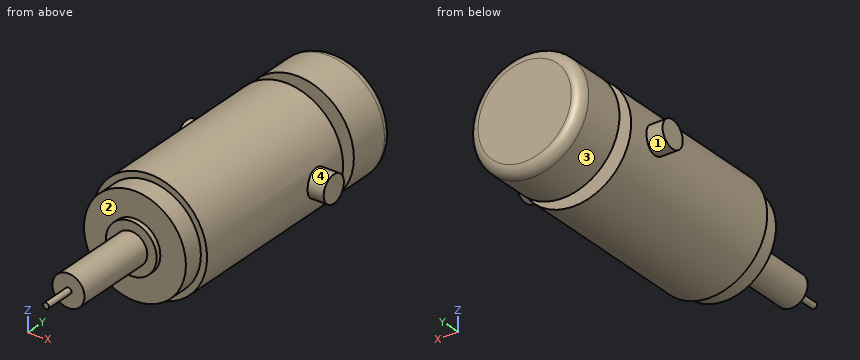
```python
from build123d import *

# Parameters (mm, degrees)
SKETCH1_R           = 28.5
BOSS_EXTRUDE1_DEPTH = 45.5
SKETCH4_R           = 25.4
BOSS_EXTRUDE4_DEPTH = 10
SKETCH5_R           = 12.65
BOSS_EXTRUDE5_DEPTH = 2.5
SKETCH2_R           = 8
BOSS_EXTRUDE2_DEPTH = 42
SKETCH6_R           = 4
BOSS_EXTRUDE6_DEPTH = 33
SKETCH7_R           = 28.25
BOSS_EXTRUDE7_DEPTH = 25.5
FILLET1_R           = 5
SKETCH3_R           = 1.5
BOSS_EXTRUDE3_DEPTH = 15
SKETCH8_R           = 6.75
BOSS_EXTRUDE8_DEPTH = 36.5


with BuildPart() as part:
    # Sketch1 → Boss-Extrude1 (new body, symmetric)
    with BuildSketch(Plane(origin=(0, 0, 0), x_dir=(1, 0, 0), z_dir=(0, 1, 0))):
        Circle(SKETCH1_R)
    extrude(amount=BOSS_EXTRUDE1_DEPTH, both=True)

    # Sketch4 → Boss-Extrude4 (add)
    with BuildSketch(Plane.XZ.offset(45.5)):
        Circle(SKETCH4_R)
    extrude(amount=BOSS_EXTRUDE4_DEPTH)

    # Sketch5 → Boss-Extrude5 (add)
    with BuildSketch(Plane.XZ.offset(55.5)):
        Circle(SKETCH5_R)
    extrude(amount=BOSS_EXTRUDE5_DEPTH)

    # Sketch2 → Boss-Extrude2 (add)
    with BuildSketch(Plane.XZ.offset(58)):
        Circle(SKETCH2_R)
    extrude(amount=BOSS_EXTRUDE2_DEPTH)

    # Sketch6 → Boss-Extrude6 (add)
    with BuildSketch(Plane(origin=(0, 45.5, 0), x_dir=(1, 0, 0), z_dir=(0, 1, 0))):
        Circle(SKETCH6_R)
    extrude(amount=BOSS_EXTRUDE6_DEPTH)

    # Sketch7 → Boss-Extrude7 (add)
    with BuildSketch(Plane(origin=(0, 78.5, 0), x_dir=(1, 0, 0), z_dir=(0, 1, 0))):
        Circle(SKETCH7_R)
    extrude(amount=-BOSS_EXTRUDE7_DEPTH)

    # Fillet1
    fillet1_edges = [part.edges().sort_by_distance(p)[0] for p in [
        (-28.25, 78.5, 0),
    ]]
    fillet(fillet1_edges, radius=FILLET1_R)

    # Sketch3 → Boss-Extrude3 (add)
    with BuildSketch(Plane.XZ.offset(100)):
        Circle(SKETCH3_R)
    extrude(amount=BOSS_EXTRUDE3_DEPTH)

    # Sketch8 → Boss-Extrude8 (add, symmetric)
    with BuildSketch(Plane(origin=(0, 0, 0), x_dir=(0, 0, -1), z_dir=(1, 0, 0))):
        with Locations((0, 28.5)):
            Circle(SKETCH8_R)
    extrude(amount=BOSS_EXTRUDE8_DEPTH, both=True)


solid = part.part
```
Check sheet for the modelled part. Datum: model origin and axes. Units: mm. Face numbers are marked on the shaded views. A direction names the side the tool comes from. Give positions to 0.01 mm unless a question says otherwise; leave off trailing zeros. Loops run counter-clockwise (first coordinate to the right, second up) from the corner with the lowest first, then second, coordinate; pieces in that order, holes last. Notation, with made-up numbers: (78, -19) - (126, -19) arc R22 ccw to (126, -13) - close; hole circle Ø7 at (63.5, 9.5). An arc over 180 degrees is marked (long way). One line per question, with ' | ' between items. Start each with the question number.
1. Cross-section at B-B, the plane y = 50.5. Enter the section's corners in (x, z).
2. Material ranges on line 1 along Y through (x, z) = (-15, 16); line 2 along Y through (x, z) = (-4.5, -10.5); line 3 along X through (y, z) = (-3, -4), recorded low to high. Write a range as [from, to].
3. Set-up check for the marked faces 1, 2, 3 and 4: record each of +Z, -Z, +X, -X, +Y, -Y from which the full face is reachable in a straight line by a thin tool's end or side.
4. Cross-section at A-A, the plane y = -32.5. Enter the section's corners in (x, z), plus the area to 3 significant figures.
5. Gauge pin test, flat ends, axial feed: pin 1 Ø2 at (y, z) = (19, 0.5) entering from -X; pin 2 Ø2 at (x, y) = (-19.5, 44.5) entering from -Z; pin 3 Ø5 at (y, z) = (-17.5, 13) entering from +X; pin 4 Ø12.5 at (x, z) = (-4.5, 5) entering from -Y. Record the tip position at first contact, or that the pin passes through.
Check result:
1) outline: circle Ø8 at (0, 0)
2) line 1: y = [-55.5, 45.5], [53, 78.5] | line 2: y = [-58, 45.5], [53, 78.5] | line 3: x = [-28.22, 28.22]
3) face 1: -X | face 2: -Y | face 3: +Y | face 4: +X
4) outline: circle Ø57 at (0, 0) | area: 2,550 mm2
5) pin 1: stops at x = -28.5 | pin 2: stops at z = -21.68 | pin 3: stops at x = 26.5 | pin 4: stops at y = -115
